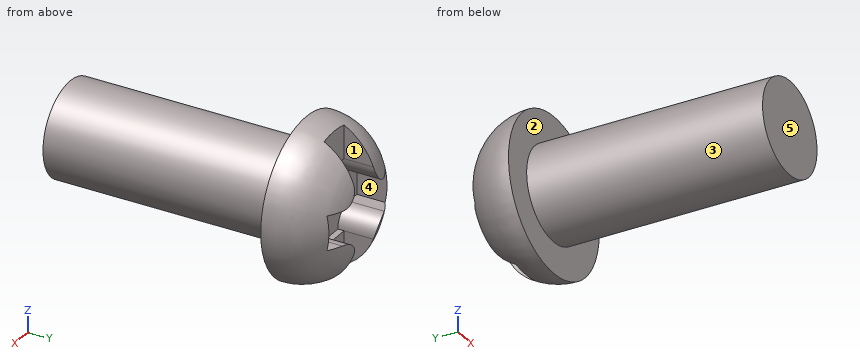
from build123d import *

# Parameters (mm, degrees)
SKETCH3_W           = 1.1
SKETCH3_H           = 4.9
CUT_EXTRUDE1_DEPTH  = 1.1
SKETCH4_W           = 3.2
SKETCH4_H           = 1.1
CUT_EXTRUDE2_DEPTH  = 4.702516225
FILLET1_R           = 0.6
CUT_EXTRUDE3_DEPTH  = 0.2
SKETCH2_R           = 1.5
BOSS_EXTRUDE1_DEPTH = 7.6


with BuildPart() as part:
    # Sketch1 → Revolve1 (revolve)
    with BuildSketch(Plane(origin=(0, 0, 0), x_dir=(0, 0, -1), z_dir=(1, 0, 0))):
        with BuildLine():
            Line((0, 2), (0, 0))
            Line((0, 0), (2.5, 0))
            ThreePointArc((2.5, 0), (1.914213562, 1.414213562), (0.5, 2))
            Line((0.5, 2), (0, 2))
        make_face()
    revolve(axis=Axis((0, 0, 0), (0, 1, 0)))

    # Sketch3 → Cut-Extrude1 (cut)
    with BuildSketch(Plane(origin=(0, 2, 0), x_dir=(1, 0, 0), z_dir=(0, 1, 0))):
        Rectangle(SKETCH3_W, SKETCH3_H)
    extrude(amount=-CUT_EXTRUDE1_DEPTH, mode=Mode.SUBTRACT)

    # Sketch4 → Cut-Extrude2 (cut, through all)
    with BuildSketch(Plane(origin=(0, 0.9, 0), x_dir=(1, 0, 0), z_dir=(0, 1, 0))):
        Rectangle(SKETCH4_W, SKETCH4_H)
    extrude(amount=CUT_EXTRUDE2_DEPTH, mode=Mode.SUBTRACT)

    # Fillet1
    fillet1_edges = [part.edges().sort_by_distance(p)[0] for p in [
        (0.55, 1.440305176, 0.55),
        (-0.55, 1.440305183, 0.55),
        (0.55, 1.440305183, -0.55),
        (-0.55, 1.440305176, -0.55),
    ]]
    fillet(fillet1_edges, radius=FILLET1_R)

    # Sketch5 → Cut-Extrude3 (cut)
    with BuildSketch(Plane(origin=(0, 0.9, 0), x_dir=(1, 0, 0), z_dir=(0, 1, 0))):
        with BuildLine():
            Line((-0.55, 1.15), (0.55, 1.15))
            ThreePointArc((0.55, 1.15), (0.725735931, 0.725735931), (1.15, 0.55))
            Line((1.15, 0.55), (1.6, 0.55))
            Line((1.6, 0.55), (1.6, -0.55))
            Line((1.6, -0.55), (1.15, -0.55))
            ThreePointArc((1.15, -0.55), (0.725735931, -0.725735931), (0.55, -1.15))
            Line((0.55, -1.15), (-0.55, -1.15))
            ThreePointArc((-0.55, -1.15), (-0.725735931, -0.725735931), (-1.15, -0.55))
            Line((-1.15, -0.55), (-1.6, -0.55))
            Line((-1.6, -0.55), (-1.6, 0.55))
            Line((-1.6, 0.55), (-1.15, 0.55))
            ThreePointArc((-1.15, 0.55), (-0.725735931, 0.725735931), (-0.55, 1.15))
        make_face()
    extrude(amount=-CUT_EXTRUDE3_DEPTH, mode=Mode.SUBTRACT)

    # Sketch2 → Boss-Extrude1 (add)
    with BuildSketch(Plane.XZ):
        with Locations(Location((0, 0, 0), (0, 0, 90))):
            Circle(SKETCH2_R)
    extrude(amount=BOSS_EXTRUDE1_DEPTH)


solid = part.part
Source: CAD feature listing. Evaluate the final solid. Frame: model axes, mm. Face numbers are marked on the shaded views. A direction names the side the tool comes from. Round coordinates to 2 decimals unless told otherwise and drop trailing zeros. Loops run counter-clockwise (first coordinate to the right, second up) from the corner with the lowest first, then second, coordinate; pieces in that order, holes last.
Q1. First-contact query: P1, Ø0.8, axis at y = 1.5, z = -2, coming from the +X side; P2, Ø2, axis at y = -3.5, z = -1, coming from the -X side; P3, Ø0.9, axis at x = -0.5, z = 1.5, coming from the +Y side. Flat tips, straight axial feed; report the tip coordinate or a pass-through.
Q2. Access query for the marked faces 1 and 2. Directions: +Z, -Z, +X, -X, +Y, -Y. A direction counts if a zero-diameter tool reaches every point of the face in a straight line with its end or side. Return the directions, or none.
Q3. Ray query, line 1 (Y direction, x = 0.8, z = -0.1); line 2 (Y direction, x = -0.4, z = 1.6); line 3 (Z direction, x = 0.4, y = 0.75). Return the intervals inside material, ascending.
Q4. Section A-A, the plane y = -2.25. Return loops of the section in (x, z), plus the area to 3 significant figures.
Q5. Mould query, pull axis X, two halves, no side actions, for the marked faces 3, 4 and 5. Classes: pulls with the +X half, pulls with the -X half, needs draft (parallel to the pull), parting line crosses it, or undercut.
Solutions:
1. P1: stops at x = 1.19
1. P2: stops at x = -1.5
1. P3: stops at y = 1.88
2. face 1: +Z, -Z, +Y
2. face 2: -Y
3. line 1: y = -7.6 to 0.7
3. line 2: y = 0 to 0.9
3. line 3: z = -2.32 to -1.15, 1.15 to 2.32
4. outline: circle Ø3 at (0, 0)
4. area: 7.07 mm2
5. face 3: parting line crosses it
5. face 4: undercut
5. face 5: needs draft
